Can you work these out from the model? Positions are in its coordinate system, mm. A direction names the side the tool comes from. Round coordinates to 2 decimals unless told otherwise and drop trailing zeros. Write each loop counter-clockwise with the first axis right and the second up, starting at its lowest first coordinate (ties: lowest second). Pieces come first, ordered by that corner, then holes.
Q1. If we section it at A-A (z = 0): Please give me the cut outline in (x, y).
Q2. I'm going to push flat-ended pins straight in: pin 1 Ø1.8 at (x, y) = (1.5, 36.5) entering from +Z; pin 2 Ø3 at (x, y) = (1.5, 4) entering from -Z; pin 3 Ø3 at (x, y) = (-0.5, 64) entering from -Z. Where does each tip first touch, or does it pass through?
Q3. If we section it at B-B (x = -1.75): Please give me the cut outline in (y, z).
Q4. Please list where these lines run through material, in increasing order: line 1 along X through (y, z) = (8, -10.5); line 2 along X through (y, z) = (62, 0); line 3 along Z through (x, y) = (6.5, 73.5).
Q5. We'd pull the mould along Y, two halves only. Please class faces 4 (the flat face through (-4.508, 53, 0)), 5 (the cylindrical face through (-11.18, 12.61, -6.35)): +Y half, -Y half, draft (parallel to the pull), parting line (faces both ways), or undercut.
Q6. For faces 1 (the cylindrical face through (11.23, 12.61, -6.35)), 2 (the flat face through (-4.508, 3, 0)), 3 (the flat face through (0, 4, 4.508)), which set-ups out of +Z, -Z, +X, -X, +Y, -Y let a thin tool reach every point of the face, with its end or its side?
Q7. If we section it at C-C (y = 12.7): Give the number of separate pieces and of enclosed holes in the cut face, plus the area to 3 significant figures.
from build123d import *

# Parameters (mm, degrees)
SKETCH1_W           = 25.4
SKETCH1_H           = 25.4
BOSS_EXTRUDE1_DEPTH = 88.9
SKETCH2_R           = 6.35
CUT_EXTRUDE1_DEPTH  = 26.4
SKETCH4_R           = 2.6035
CUT_EXTRUDE2_DEPTH  = 89.9


with BuildPart() as part:
    # Sketch1 → Boss-Extrude1 (new body)
    with BuildSketch(Plane(origin=(0, 0, 0), x_dir=(1, 0, 0), z_dir=(0, 1, 0))):
        Rectangle(SKETCH1_W, SKETCH1_H)
    extrude(amount=BOSS_EXTRUDE1_DEPTH)

    # Sketch2 → Cut-Extrude1 (cut, through all)
    with BuildSketch(Plane(origin=(12.7, 0, 0), x_dir=(0, 0, -1), z_dir=(1, 0, 0))):
        with Locations((0, 12.7)):
            Circle(SKETCH2_R)
    extrude(amount=-CUT_EXTRUDE1_DEPTH, mode=Mode.SUBTRACT)

    # Sketch4 → Cut-Extrude2 (cut, through all)
    with BuildSketch(Plane.XZ):
        Circle(SKETCH4_R)
        with BuildLine():
            Line((-3.2385, 12.7), (3.2385, 12.7))
            Line((3.2385, 12.7), (3.2385, 10.218485055))
            ThreePointArc((3.2385, 10.218485055), (3.387289755, 9.85927481), (3.7465, 9.710485055))
            Line((3.7465, 9.710485055), (6.9215, 9.710485055))
            ThreePointArc((6.9215, 9.710485055), (7.390830803, 9.396888238), (7.280710245, 8.84327481))
            Line((7.280710245, 8.84327481), (2.945935435, 4.5085))
            Line((2.945935435, 4.5085), (-2.945935435, 4.5085))
            Line((-2.945935435, 4.5085), (-7.280710245, 8.84327481))
            ThreePointArc((-7.280710245, 8.84327481), (-7.390830803, 9.396888238), (-6.9215, 9.710485055))
            Line((-6.9215, 9.710485055), (-3.7465, 9.710485055))
            ThreePointArc((-3.7465, 9.710485055), (-3.387289755, 9.85927481), (-3.2385, 10.218485055))
            Line((-3.2385, 10.218485055), (-3.2385, 12.7))
        make_face()
        with BuildLine():
            Line((12.7, 3.2385), (12.7, -3.2385))
            Line((12.7, -3.2385), (10.218485055, -3.2385))
            ThreePointArc((10.218485055, -3.2385), (9.85927481, -3.387289755), (9.710485055, -3.7465))
            Line((9.710485055, -3.7465), (9.710485055, -6.9215))
            ThreePointArc((9.710485055, -6.9215), (9.396888238, -7.390830803), (8.84327481, -7.280710245))
            Line((8.84327481, -7.280710245), (4.5085, -2.945935435))
            Line((4.5085, -2.945935435), (4.5085, 2.945935435))
            Line((4.5085, 2.945935435), (8.84327481, 7.280710245))
            ThreePointArc((8.84327481, 7.280710245), (9.396888238, 7.390830803), (9.710485055, 6.9215))
            Line((9.710485055, 6.9215), (9.710485055, 3.7465))
            ThreePointArc((9.710485055, 3.7465), (9.85927481, 3.387289755), (10.218485055, 3.2385))
            Line((10.218485055, 3.2385), (12.7, 3.2385))
        make_face()
        with BuildLine():
            Line((3.2385, -12.7), (-3.2385, -12.7))
            Line((-3.2385, -12.7), (-3.2385, -10.218485055))
            ThreePointArc((-3.2385, -10.218485055), (-3.387289755, -9.85927481), (-3.7465, -9.710485055))
            Line((-3.7465, -9.710485055), (-6.9215, -9.710485055))
            ThreePointArc((-6.9215, -9.710485055), (-7.390830803, -9.396888238), (-7.280710245, -8.84327481))
            Line((-7.280710245, -8.84327481), (-2.945935435, -4.5085))
            Line((-2.945935435, -4.5085), (2.945935435, -4.5085))
            Line((2.945935435, -4.5085), (7.280710245, -8.84327481))
            ThreePointArc((7.280710245, -8.84327481), (7.390830803, -9.396888238), (6.9215, -9.710485055))
            Line((6.9215, -9.710485055), (3.7465, -9.710485055))
            ThreePointArc((3.7465, -9.710485055), (3.387289755, -9.85927481), (3.2385, -10.218485055))
            Line((3.2385, -10.218485055), (3.2385, -12.7))
        make_face()
        with BuildLine():
            Line((-12.7, -3.2385), (-12.7, 3.2385))
            Line((-12.7, 3.2385), (-10.218485055, 3.2385))
            ThreePointArc((-10.218485055, 3.2385), (-9.85927481, 3.387289755), (-9.710485055, 3.7465))
            Line((-9.710485055, 3.7465), (-9.710485055, 6.9215))
            ThreePointArc((-9.710485055, 6.9215), (-9.396888238, 7.390830803), (-8.84327481, 7.280710245))
            Line((-8.84327481, 7.280710245), (-4.5085, 2.945935435))
            Line((-4.5085, 2.945935435), (-4.5085, -2.945935435))
            Line((-4.5085, -2.945935435), (-8.84327481, -7.280710245))
            ThreePointArc((-8.84327481, -7.280710245), (-9.396888238, -7.390830803), (-9.710485055, -6.9215))
            Line((-9.710485055, -6.9215), (-9.710485055, -3.7465))
            ThreePointArc((-9.710485055, -3.7465), (-9.85927481, -3.387289755), (-10.218485055, -3.2385))
            Line((-10.218485055, -3.2385), (-12.7, -3.2385))
        make_face()
    extrude(amount=-CUT_EXTRUDE2_DEPTH, mode=Mode.SUBTRACT)


solid = part.part
A:
1. outline: (-4.51, 0) - (-2.6, 0) - (-2.6, 6.35) - (-4.51, 6.35) - close; (-4.51, 19.05) - (-2.6, 19.05) - (-2.6, 88.9) - (-4.51, 88.9) - close; (2.6, 0) - (4.51, 0) - (4.51, 6.35) - (2.6, 6.35) - close; (2.6, 19.05) - (4.51, 19.05) - (4.51, 88.9) - (2.6, 88.9) - close
2. pin 1: stops at z = 4.51
2. pin 2: stops at z = -4.56
2. pin 3: stops at z = -4.51
3. outline: (0, -4.51) - (8.23, -4.51) arc R6.35 cw to (6.65, -1.93) - (0, -1.93) - close; (0, 1.93) - (6.65, 1.93) arc R6.35 cw to (8.23, 4.51) - (0, 4.51) - close; (17.17, -4.51) - (88.9, -4.51) - (88.9, -1.93) - (18.75, -1.93) arc R6.35 cw to start; (17.17, 4.51) arc R6.35 cw to (18.75, 1.93) - (88.9, 1.93) - (88.9, 4.51) - close
4. line 1: x = -12.7 to -3.24, 3.24 to 12.7
4. line 2: x = -4.51 to -2.6, 2.6 to 4.51
4. line 3: z = -12.7 to -9.71, -8.06 to -4.94, 4.94 to 8.06, 9.71 to 12.7
5. face 4: draft
5. face 5: undercut
6. face 1: +X, -X
6. face 2: -X, +Y, -Y
6. face 3: +Z, +Y, -Y
7. separate pieces: 4
7. enclosed holes: 0
7. area: 193 mm2
